For this review, take the finished solid that the model builds, in its own axes (mm). A direction names the side the tool comes from. Coordinates: 2 decimals unless noted, no trailing zeros. Write each loop counter-clockwise with the first axis right and the second up, starting at its lowest first coordinate (ties: lowest second). Pieces come first, ordered by that corner, then holes.
1) For faces 5 (the face through (-0.738, 15.024, -6.203)), 6 (the face through (0, -4, 0)), 7 (the face through (6.35, -11, 0)), list the 3-axis set-ups (+Z, -Z, +X, -X, +Y, -Y) from which the entire face can be reached by the end or side of a thin tool; tool diameter is ignored.
2) We need section B-B on x = 5.75. Write out the cut boundary in (y, z), then the cut area to 3 significant figures.
3) To check wall thickness, follow line 1 along Z through (x, y) = (-0.5, 12); line 2 along Y through (x, z) = (0.8, 0); line 3 along X through (y, z) = (21.5, 4). State the ranges of each line that lie inside material, in increasing order.
4) We need section C-C on y = 16.5. Write out the cut boundary in (x, z).
5) We need section D-D on y = 8. Write out the cut boundary in (x, z), then the cut area to 3 significant figures.
6) Insertion check: P1, Ø1.6, axis at x = -0.5, z = -5.5, coming from the +Y side; P2, Ø1.2, axis at x = -0.44, z = 5.27, coming from the +Y side; P3, Ø4, axis at y = -9, z = -3, coming from the -X side; P4, Ø4, axis at y = -6.477, z = 0, coming from the -X side. Each pin has a flat end and moves straight along its axis. Give the tip position at first contact, or say it passes through.
7) We need section A-A on z = 0. Write out the cut boundary in (x, y).
8) Mouldability with a two-part tool opening along Z and no side actions: class faces 1 (the face through (3, -12.7, 0)), 2 (the face through (5, 9, 12.7)), 3 (the face through (-3.238, 22, 0)), 4 (the face through (8, 22, -7.823)) as pulls with the +Z half, pulls with the -Z half, needs draft (parallel to the pull), parting line crosses it, or undercut.
from build123d import *

# Parameters (mm, degrees)
PROFILE_W               = 12.7
PROFILE_H               = 22.86
PROFILE_W_2             = 6.35
PROFILE_H_2             = 12.7
BOSS_EXTRUDE1_DEPTH     = 12.7
CUT_EXTRUDE1_DEPTH      = 27.910817528
CUT_EXTRUDE1_DEPTH_BACK = 27.910817528
SCREWHOLE_R             = 2.159
CUT_EXTRUDE2_START      = -4.064
SKETCH3_R               = 3.683
SKETCH3_R_2             = 2.159
CUT_EXTRUDE2_DEPTH      = 4.064
SKETCH4_W               = 25.4
SKETCH4_H               = 12.7
BOSS_EXTRUDE2_DEPTH     = 12.7
SKETCH6_W               = 19.177
SKETCH6_H               = 15.6464
CUT_EXTRUDE3_DEPTH      = 1.5748
SKETCH9_W               = 13.589
SKETCH9_H               = 15.6464
CUT_EXTRUDE5_DEPTH      = 1.143
SKETCH7_R               = 0.9779
CUT_EXTRUDE6_DEPTH      = 12.7
FILLET1_R               = 19.05
FILLET2_R               = 5.08


with BuildPart() as part:
    # Profile → Boss-Extrude1 (new, symmetric)
    with BuildSketch(Plane.XY):
        with Locations((0, 11.43)):
            Rectangle(PROFILE_W, PROFILE_H)
        with Locations((3.175, -6.35)):
            Rectangle(PROFILE_W_2, PROFILE_H_2)
    extrude(amount=BOSS_EXTRUDE1_DEPTH, both=True)

    # ScrewHole → Cut-Extrude1 (cut, two sides: drawn at the far end of the back side and taken through both)
    with BuildSketch(Plane.ZY.offset(-CUT_EXTRUDE1_DEPTH_BACK)):
        with Locations(Location((0, -6.477, 0), (0, 0, 270))):
            Circle(SCREWHOLE_R)
    extrude(amount=CUT_EXTRUDE1_DEPTH + CUT_EXTRUDE1_DEPTH_BACK, mode=Mode.SUBTRACT)

    # Sketch3 → Cut-Extrude2 (cut)
    with BuildSketch(Plane(origin=(6.35, 0, 0), x_dir=(0, 0, -1), z_dir=(1, 0, 0)).offset(CUT_EXTRUDE2_START)):
        with Locations(Location((0, -6.477, 0), (0, 0, 90))):
            Circle(SKETCH3_R)
        with Locations(Location((0, -6.477, 0), (0, 0, 270))):
            Circle(SKETCH3_R_2, mode=Mode.SUBTRACT)
    extrude(amount=CUT_EXTRUDE2_DEPTH, mode=Mode.SUBTRACT)

    # Sketch4 → Boss-Extrude2 (add)
    with BuildSketch(Plane(origin=(6.35, 0, 0), x_dir=(0, 0, -1), z_dir=(1, 0, 0))):
        with Locations((0, 16.51)):
            Rectangle(SKETCH4_W, SKETCH4_H)
    extrude(amount=BOSS_EXTRUDE2_DEPTH)

    # Sketch6 → Cut-Extrude3 (cut)
    with BuildSketch(Plane(origin=(0, 22.86, 0), x_dir=(1, 0, 0), z_dir=(0, 1, 0))):
        with Locations((6.35, 0)):
            Rectangle(SKETCH6_W, SKETCH6_H)
    extrude(amount=-CUT_EXTRUDE3_DEPTH, mode=Mode.SUBTRACT)

    # Sketch9 → Cut-Extrude5 (cut)
    with BuildSketch(Plane(origin=(0, 21.2852, 0), x_dir=(1, 0, 0), z_dir=(0, 1, 0))):
        with Locations((9.144, 0)):
            Rectangle(SKETCH9_W, SKETCH9_H)
    extrude(amount=-CUT_EXTRUDE5_DEPTH, mode=Mode.SUBTRACT)

    # Sketch7 → Cut-Extrude6 (cut)
    with BuildSketch(Plane(origin=(0, 21.2852, 0), x_dir=(1, 0, 0), z_dir=(0, 1, 0))):
        with Locations(Location((-0.4445, -5.2705, 0), (0, 0, 90))):
            Circle(SKETCH7_R)
        with Locations(Location((-0.4445, 5.2705, 0), (0, 0, 90))):
            Circle(SKETCH7_R)
    extrude(amount=-CUT_EXTRUDE6_DEPTH, mode=Mode.SUBTRACT)

    # Fillet1
    # the kernel refuses this fillet: 19.05 mm, written as the material it adds along each edge
    with BuildSketch(Plane(origin=(6.35, 10.16, -12.7), x_dir=(0, -1, 0), z_dir=(0, 0, 1))) as fillet1_piece_1_section:
        with BuildLine():
            CenterArc((17.960512242, 19.05), FILLET1_R, 199.471220634, 70.528779366)
            Line((0, 12.7), (0, 0))
            Line((0, 0), (17.960512242, 0))
        make_face()
    fillet1_piece_1 = extrude(amount=25.4, mode=Mode.PRIVATE)
    fillet1_piece_1 = fillet1_piece_1 - Plane(origin=(6.35, -6.477, 0), x_dir=(0, 1, 0), z_dir=(-1, 0, 0)) * Cylinder(3.683, 123, mode=Mode.PRIVATE)
    add(fillet1_piece_1)

    # Fillet2
    fillet2_edges = [part.edges().sort_by_distance(p)[0] for p in [
        (-6.35, 11.43, 12.7),
        (19.05, 16.51, 12.7),
        (19.05, 16.51, -12.7),
        (-6.35, 11.43, -12.7),
    ]]
    fillet(fillet2_edges, radius=FILLET2_R)


solid = part.part
Result:
1. face 5: +Y
1. face 6: +Z, -Z, -X, -Y
1. face 7: +Z, -Z, +X, -Y
2. outline: (-12.7, -12.7) - (22.86, -12.7) - (22.86, -7.82) - (20.14, -7.82) - (20.14, 7.82) - (22.86, 7.82) - (22.86, 12.7) - (-12.7, 12.7) - close; hole circle Ø7.37 at (-6.48, 0)
2. area: 818 mm2
3. line 1: z = -12.7 to -6.25, -4.29 to 4.29, 6.25 to 12.7
3. line 2: y = -12.7 to -8.64, -4.32 to 21.29
3. line 3: x = -6.35 to -3.24, 15.94 to 19.05
4. outline: (-6.35, -7.62) arc R5.08 ccw to (-1.27, -12.7) - (13.97, -12.7) arc R5.08 ccw to (19.05, -7.62) - (19.05, 7.62) arc R5.08 ccw to (13.97, 12.7) - (-1.27, 12.7) arc R5.08 ccw to (-6.35, 7.62) - close; hole circle Ø1.96 at (-0.44, -5.27); hole circle Ø1.96 at (-0.44, 5.27)
5. outline: (-6.35, -7.62) arc R5.08 ccw to (-1.27, -12.7) - (13.97, -12.7) arc R5.08 ccw to (14.76, -12.64) - (14.76, 12.64) arc R5.08 ccw to (13.97, 12.7) - (-1.27, 12.7) arc R5.08 ccw to (-6.35, 7.62) - close
5. area: 525 mm2
6. P1: stops at y = 21.29
6. P2: stops at y = 8.59
6. P3: stops at x = 0
6. P4: passes through
7. outline: (-6.35, 0) - (0, 0) - (0, -4.32) - (2.29, -4.32) - (2.29, -2.79) - (7.02, -2.79) arc R19.05 cw to (19.05, 10.16) - (19.05, 22.86) - (15.94, 22.86) - (15.94, 20.14) - (2.35, 20.14) - (2.35, 21.29) - (-3.24, 21.29) - (-3.24, 22.86) - (-6.35, 22.86) - close; (0, -12.7) - (6.35, -12.7) - (6.35, -10.16) - (2.29, -10.16) - (2.29, -8.64) - (0, -8.64) - close
8. face 1: needs draft
8. face 2: pulls with the +Z half
8. face 3: undercut
8. face 4: undercut
